from build123d import *

# Parameters (mm, degrees)
SKETCH2_R          = 3.25
CUT_EXTRUDE1_DEPTH = 74.188113789
SKETCH3_R          = 2.1
CUT_EXTRUDE2_DEPTH = 20
CIRPATTERN1_COUNT  = 6
CHAMFER1_SIZE      = 1
CUT_EXTRUDE3_START = -6
CUT_EXTRUDE3_DEPTH = 6


with BuildPart() as part:
    # Sketch1 → Revolve1 (revolve)
    with BuildSketch(Plane.XY, mode=Mode.PRIVATE) as revolve1_sk:
        Polygon((0, 0), (0, 27.5), (45, 27.5), (45, 16), (62, 16), (62, 0), align=None)
    revolve(revolve1_sk.sketch.rotate(Axis((0, 0, 0), (1, 0, 0)), 90), axis=Axis((0, 0, 0), (1, 0, 0)))

    # Sketch2 → Cut-Extrude1 (cut, through all)
    with BuildSketch(Plane.ZY):
        with Locations((-7, 7)):
            Circle(SKETCH2_R)
        with Locations(Location((7, 7, 0), (0, 0, 180))):
            Circle(SKETCH2_R)
        with Locations((7, -7)):
            Circle(SKETCH2_R)
        with Locations(Location((-7, -7, 0), (0, 0, 180))):
            Circle(SKETCH2_R)
    extrude(amount=-CUT_EXTRUDE1_DEPTH, mode=Mode.SUBTRACT)

    # Sketch3 → Cut-Extrude2 (cut)
    with BuildSketch(Plane(origin=(45, 0, 0), x_dir=(0, 0, -1), z_dir=(1, 0, 0))):
        with Locations((0, 22)):
            Circle(SKETCH3_R)
    cut_extrude2 = extrude(amount=-CUT_EXTRUDE2_DEPTH, mode=Mode.SUBTRACT)

    # CirPattern1: Cut-Extrude2 ×6 about axis
    cirpattern1_axis = Axis((0, 0, 0), (1, 0, 0))
    for i in range(1, CIRPATTERN1_COUNT):
        add(cut_extrude2.rotate(cirpattern1_axis, i * 360 / CIRPATTERN1_COUNT), mode=Mode.SUBTRACT)

    # Chamfer1
    chamfer1_edges = [part.edges().sort_by_distance(p)[0] for p in [
        (0, -7, -3.75),
        (0, -7, 3.75),
        (0, 7, 10.25),
        (0, 7, -10.25),
        (45, 0, -27.5),
        (0, 0, -27.5),
    ]]
    chamfer(chamfer1_edges, length=CHAMFER1_SIZE)

    # Sketch4 → Cut-Extrude3 (cut)
    with BuildSketch(Plane.ZY.offset(CUT_EXTRUDE3_START)):
        with BuildLine():
            Line((-18.874586088, 20), (18.874586088, 20))
            ThreePointArc((18.874586088, 20), (27.5, 0), (18.874586088, -20))
            Line((18.874586088, -20), (-18.874586088, -20))
            ThreePointArc((-18.874586088, -20), (-27.5, 0), (-18.874586088, 20))
        make_face()
    extrude(amount=CUT_EXTRUDE3_DEPTH, mode=Mode.SUBTRACT)


solid = part.part
Geometry: final body of the model. Coordinates: model frame, mm. A direction names the side the tool comes from. Round coordinates to 2 decimals unless told otherwise and drop trailing zeros. Loops run counter-clockwise (first coordinate to the right, second up) from the corner with the lowest first, then second, coordinate; pieces in that order, holes last.
Q1. Section A-A on x = 46. Return loops of the section in (y, z).
Q2. Section B-B on z = 0. Return loops of the section in (x, y), plus the area to 3 significant figures.
Q3. Pull-direction query (Y, two-part tool) for faces 1 (the cylindrical face through (33.608, -10.222, -6.577)), 2 (the cylindrical face through (22.8, -8.26, 26.23)), 3 (the conical face through (0.2, 26.7, -0.3)), 4 (the flat face through (45, 17, 0)); classes: released by +Y, released by -Y, zero draft, split by the parting line, or undercut.
Q4. Material intervals for L1, parallel to Y at x = 35.75, z = 0; L2, parallel to X at y = -22.5, z = 8.5; L3, parallel to X at y = -16, z = -2.5, sorted ascending.
Q5. Access query for faces 5 (the flat face through (6, 0, 0)), 6 (the cylindrical face through (35.14, 9.58, -20.6)), 7 (the flat face through (0, 22, 0)). Directions: +Z, -Z, +X, -X, +Y, -Y. A direction counts if a zero-diameter tool reaches every point of the face in a straight line with its end or side. Return the directions, or none.
Q6. Section C-C on x = 33. State how many separate pieces and enclosed holes the cut face has, plus the area to 3 significant figures.
Q7. Pin query (flat end, axial travel): P1, Ø6.5, axis at y = -11, z = -19.05, coming from the -X side; P2, Ø2, axis at y = 13, z = -21.5, coming from the +X side; P3, Ø2.5, axis at y = 11, z = -19.05, coming from the +X side. Return the tip coordinate at first contact, or that it passes through.
Q8. Section D-D on x = 10. Return loops of the section in (y, z).
Evaluation:
1. outline: circle Ø32 at (0, 0); hole circle Ø6.5 at (-7, -7); hole circle Ø6.5 at (-7, 7); hole circle Ø6.5 at (7, -7); hole circle Ø6.5 at (7, 7)
2. outline: (0, -26.5) - (1, -27.5) - (44, -27.5) - (45, -26.5) - (45, -24.1) - (25, -24.1) - (25, -19.9) - (45, -19.9) - (45, -16) - (62, -16) - (62, 16) - (45, 16) - (45, 19.9) - (25, 19.9) - (25, 24.1) - (45, 24.1) - (45, 26.5) - (44, 27.5) - (1, 27.5) - (0, 26.5) - (0, 20) - (6, 20) - (6, -20) - (0, -20) - close
2. area: 2,610 mm2
3. face 1: undercut
3. face 2: split by the parting line
3. face 3: released by +Y
3. face 4: zero draft
4. L1: y = -27.5 to -24.1, -19.9 to 19.9, 24.1 to 27.5
4. L2: x = 0 to 45
4. L3: x = 6 to 45
5. face 5: +Z, -Z, -X
5. face 6: +X
5. face 7: +Z, -Z, -X, +Y, -Y
6. separate pieces: 1
6. enclosed holes: 10
6. area: 2,160 mm2
7. P1: stops at x = 6
7. P2: stops at x = 45
7. P3: stops at x = 25
8. outline: circle Ø55 at (0, 0); hole circle Ø6.5 at (-7, -7); hole circle Ø6.5 at (-7, 7); hole circle Ø6.5 at (7, -7); hole circle Ø6.5 at (7, 7)
